Autodesk Inventor part; units mm, degrees
ref_plane "YZ Plane" through (0, 0, 0) normal (1, 0, 0) x (0, 1, 0)
ref_plane "XZ Plane" through (0, 0, 0) normal (0, 1, 0) x (-1, 0, 0)
ref_plane "XY Plane" through (0, 0, 0) normal (0, 0, 1) x (1, 0, 0)
sketch "Sketch1" plane through (0, 0, 0) normal (0, 0, 1) x (1, 0, 0)
  line L0 (0.866, 0) -> (0.433, -0.75)
  line L1 (0.433, -0.75) -> (-0.433, -0.75)
  line L2 (-0.433, -0.75) -> (-0.866, 0)
  line L3 (-0.866, 0) -> (-0.433, 0.75)
  line L4 (-0.433, 0.75) -> (0.433, 0.75)
  line L5 (0.433, 0.75) -> (0.866, 0)
  point P0 (0, 0)
  point P1 (0, 0)
  point P2 (0, 0.75)
  dimension "d3" = 0.75
extrude "Extrusion1" add sketch "Sketch1" against normal blind 10
properties part number "P88041_Wheel_Hex_Pin_C"
The model under review builds one solid part; all positions refer to its coordinate system, in mm. Give positions to 0.01 mm unless a question says otherwise; leave off trailing zeros. Order: outer loops, then holes, each group sorted by start corner. A loop starts at its lowest first (then second) coordinate and runs counter-clockwise, first axis right, second up. Notation, with made-up numbers: (70, -18) -> (98, -18) arc R17 cw to (98, -10) -> close; hole circle Ø11 at (8.25, 89). An arc over 180 degrees is marked (long way). Write item = value, one per line. Start each with the question number.
(1) For L1, parallel to X at y = 0.15, z = -3.75; L2, parallel to Y at x = -0.5, z = -6; L3, parallel to Y at x = -0.7, z = -7, list the stretches that pass through material, from the lowest coordinate up. Write a range as from..to.
(2) Take a section at A-A (z = -3.25). Write out the cut boundary in (x, y), plus the area to 3 significant figures.
(3) Take a section at B-B (y = 0.6). Write out the cut boundary in (x, z), plus the area to 3 significant figures.
(4) Take a section at C-C (x = -0.7). Write out the cut boundary in (y, z), plus the area to 3 significant figures.
Returned:
q1.L1 = -0.78..0.78
q1.L2 = -0.63..0.63
q1.L3 = -0.29..0.29
q2.outline = (-0.87, 0) -> (-0.43, -0.75) -> (0.43, -0.75) -> (0.87, 0) -> (0.43, 0.75) -> (-0.43, 0.75) -> close
q2.area = 1.95 mm²
q3.outline = (-0.52, -10) -> (0.52, -10) -> (0.52, 0) -> (-0.52, 0) -> close
q3.area = 10.4 mm²
q4.outline = (-0.29, -10) -> (0.29, -10) -> (0.29, 0) -> (-0.29, 0) -> close
q4.area = 5.75 mm²
